from build123d import *

# Parameters (mm, degrees)
SKETCH2_R           = 4.5
BOSS_EXTRUDE1_DEPTH = 1.5
SKETCH3_R           = 2.5
BOSS_EXTRUDE2_DEPTH = 25
CHAMFER1_SIZE       = 0.1
CHAMFER2_SIZE       = 0.75
CHAMFER2_SIZE2      = 0.3
CUT_EXTRUDE1_DEPTH  = 3
CHAMFER3_SIZE       = 0.3


with BuildPart() as part:
    # Sketch2 → Boss-Extrude1 (new body)
    with BuildSketch(Plane(origin=(0, 0, 0), x_dir=(1, 0, 0), z_dir=(0, 1, 0))):
        with Locations(Location((0, 0, 0), (0, 0, 270))):
            Circle(SKETCH2_R)
    extrude(amount=BOSS_EXTRUDE1_DEPTH)

    # Sketch3 → Boss-Extrude2 (add)
    with BuildSketch(Plane(origin=(0, 1.5, 0), x_dir=(1, 0, 0), z_dir=(0, 1, 0))):
        with Locations(Location((0, 0, 0), (0, 0, 270))):
            Circle(SKETCH3_R)
    extrude(amount=BOSS_EXTRUDE2_DEPTH)

    # Chamfer1
    chamfer1_edges = [part.edges().sort_by_distance(p)[0] for p in [
        (0, 1.5, -2.5),
    ]]
    chamfer(chamfer1_edges, length=CHAMFER1_SIZE)

    # Chamfer2
    chamfer2_edges = [part.edges().sort_by_distance(p)[0] for p in [
        (0, 0, -4.5),
    ]]
    chamfer2_side = [part.faces().sort_by_distance(p)[0] for p in [
        (0, 0, 0),
    ]]
    chamfer(chamfer2_edges, length=CHAMFER2_SIZE, length2=CHAMFER2_SIZE2, reference=chamfer2_side[0])

    # Sketch4 → Cut-Extrude1 (cut)
    with BuildSketch(Plane.XZ):
        Polygon((-0.422737578, 1.679670486), (-1.6660061, 0.473733761), (-1.243268521, -1.205936725), (0.422737578, -1.679670486), (1.6660061, -0.473733761), (1.243268521, 1.205936725), align=None)
    extrude(amount=-CUT_EXTRUDE1_DEPTH, mode=Mode.SUBTRACT)

    # Chamfer3
    chamfer3_edges = [part.edges().sort_by_distance(p)[0] for p in [
        (0, 26.5, -2.5),
    ]]
    chamfer(chamfer3_edges, length=CHAMFER3_SIZE)


solid = part.part
Check sheet for the modelled part. Datum: model origin and axes. Units: mm. A direction names the side the tool comes from. Coordinates: 2 decimals unless noted, no trailing zeros. Write each loop counter-clockwise with the first axis right and the second up, starting at its lowest first coordinate (ties: lowest second). Pieces come first, ordered by that corner, then holes. Notation, with made-up numbers: M 3.5,78 L 8.5,78 A12 cw 8.5,82 Z; hole C 54,-3.75 d8. An arc over 180 degrees is marked long. Answer as CSV lines item,"result".
Q1. Cross-section at B-B (z = 0). Record the boundary of the cut face in (x, y), then the cut area to 3 significant figures.
Check result:
outline,"M -4.5,0.3 L -3.75,0 L -1.55,0 L -1.55,3 L 1.55,3 L 1.55,0 L 3.75,0 L 4.5,0.3 L 4.5,1.5 L 2.6,1.5 L 2.5,1.6 L 2.5,26.2 L 2.2,26.5 L -2.2,26.5 L -2.5,26.2 L -2.5,1.6 L -2.6,1.5 L -4.5,1.5 Z"
area,"129 mm^2"
Q2. Mould release check, pull along X, two halves, no side actions. Record for faces 4 (the face through (-0.42, 1.48, -1.44)), 5 (the face through (-2.44, 13.73, -0.54)), 6 (the face through (0, 0, 2)), 7 (the face through (-1.46, 1.48, -0.35)): released by +X, released by -X, zero draft, split by the parting line, or undercut.
Check result:
face 4,"undercut"
face 5,"split by the parting line"
face 6,"zero draft"
face 7,"undercut"
Q3. Set-up check for faces 1 (the face through (0.42, 1.48, 1.44)), 2 (the face through (-2, 1.5, 2)), 3 (the face through (0, 26.5, 0)): record each of +Z, -Z, +X, -X, +Y, -Y from which the full face is reachable in a straight line by a thin tool's end or side.
Check result:
face 1,"-Y"
face 2,"+Y"
face 3,"+Z, -Z, +X, -X, +Y"
Q4. Material ranges on probe 1 along Y at (x, z) = (-2.25, 2); probe 2 along X at (y, z) = (10.25, 0); probe 3 along Y at (x, z) = (-0.5, -0.25), recorded low to high. Write a range as from..to.
Check result:
probe 1,"0..1.5"
probe 2,"-2.5..2.5"
probe 3,"3..26.5"
Q5. Cross-section at A-A (y = 16). Record the boundary of the cut face in (x, z).
Check result:
outline,"C 0,0 d5"
Q6. Cross-section at C-C (x = 0). Record the boundary of the cut face in (y, z).
Check result:
outline,"M 0,-3.75 L 0.3,-4.5 L 1.5,-4.5 L 1.5,-2.6 L 1.6,-2.5 L 26.2,-2.5 L 26.5,-2.2 L 26.5,2.2 L 26.2,2.5 L 1.6,2.5 L 1.5,2.6 L 1.5,4.5 L 0.3,4.5 L 0,3.75 L 0,1.56 L 3,1.56 L 3,-1.56 L 0,-1.56 Z"
Q7. Go/stop test with flat-tipped pins: pin 1 (4 mm diameter, centred on x = -3, z = -3, fed in from +Y); pin 2 (5 mm diameter, centred on x = -1.5, y = 23, fed in from -Z); pin 3 (4 mm diameter, centred on y = 13, z = -1.5, fed in from +X). Record where each tip stops, or that it passes through.
Check result:
pin 1,"y = 26.46"
pin 2,"z = -2.5"
pin 3,"x = 2.5"
